```python
from build123d import *

# Parameters (mm, degrees)
SKETCH_1_R               = 17.5
EXTRUDE_1_DEPTH          = 25
EXTRUDE_2_DEPTH          = 9
SKETCH_3_R               = 9
EXTRUDE_3_DEPTH          = 3
CUT_EXTRUDE_1_DEPTH      = 49.736536602
CUT_EXTRUDE_1_DEPTH_BACK = 49.736536602
SKETCH_4_W               = 40.777628878
SKETCH_4_H               = 3
CUT_EXTRUDE_2_DEPTH      = 66.193941436
CUT_EXTRUDE_2_DEPTH_BACK = 66.193941436
SKETCH_5_R               = 10
CUT_EXTRUDE_3_REACH      = 56.215
SKETCH_6_R               = 5.5
HOLE_WIZARD_M10_1_D      = 8.5
SKETCH_9_W               = 16
SKETCH_9_H               = 50
EXTRUDE_4_DEPTH          = 41
SKETCH_10_W              = 82
SKETCH_10_H              = 10
EXTRUDE_5_DEPTH          = 8
EXTRUDE_6_DEPTH          = 4
EXTRUDE_7_DEPTH          = 20
SKETCH_13_R              = 14
CUT_EXTRUDE_4_DEPTH      = 3
SKETCH_14_R              = 7.5
CUT_EXTRUDE_5_DEPTH      = 153.663027613


with BuildPart() as part:
    # Sketch 1 → Extrude 1 (new, symmetric)
    with BuildSketch(Plane.XY):
        Circle(SKETCH_1_R)
    extrude(amount=EXTRUDE_1_DEPTH, both=True)

    # Sketch 2 → Extrude 2 (add, symmetric)
    with BuildSketch(Plane(origin=(0, 0, 0), x_dir=(1, 0, 0), z_dir=(0, 1, 0))):
        with BuildLine():
            Line((0, -13), (-25, -13))
            ThreePointArc((-25, -13), (-38, 0), (-25, 13))
            Line((-25, 13), (0, 13))
            ThreePointArc((0, 13), (13, 0), (0, -13))
        make_face()
    extrude(amount=EXTRUDE_2_DEPTH, both=True)

    # Sketch 3 → Extrude 3 (add)
    with BuildSketch(Plane(origin=(0, 9, 0), x_dir=(1, 0, 0), z_dir=(0, 1, 0))):
        with Locations(Location((-25, 0, 0), (0, 0, 270))):
            Circle(SKETCH_3_R)
    extrude(amount=EXTRUDE_3_DEPTH)

    # Sketch 4 → Cut-Extrude 1 (cut, two sides: drawn at the far end of the back side and taken through both)
    with BuildSketch(Plane.XY.offset(-CUT_EXTRUDE_1_DEPTH_BACK)):
        with Locations((-20.388814439, 0)):
            Rectangle(SKETCH_4_W, SKETCH_4_H)
    extrude(amount=CUT_EXTRUDE_1_DEPTH + CUT_EXTRUDE_1_DEPTH_BACK, mode=Mode.SUBTRACT)

    # Sketch 5 → Cut-Extrude 2 (cut, two sides: drawn at the far end of the back side and taken through both)
    with BuildSketch(Plane.XY.offset(25).offset(-CUT_EXTRUDE_2_DEPTH_BACK)):
        Circle(SKETCH_5_R)
    extrude(amount=CUT_EXTRUDE_2_DEPTH + CUT_EXTRUDE_2_DEPTH_BACK, mode=Mode.SUBTRACT)

    # Sketch 6 → Cut-Extrude 3 (cut, up to next)
    with BuildSketch(Plane(origin=(0, 12, 0), x_dir=(1, 0, 0), z_dir=(0, 1, 0)), mode=Mode.PRIVATE) as cut_extrude_3_sk1:
        with Locations(Location((-25, 0, 0), (0, 0, 270))):
            Circle(SKETCH_6_R)
    cut_extrude_3_tool1 = extrude(cut_extrude_3_sk1.sketch, amount=-CUT_EXTRUDE_3_REACH, mode=Mode.PRIVATE) & part.part
    add(cut_extrude_3_tool1.solids().sort_by_distance((-25, 12, 0))[0], mode=Mode.SUBTRACT)

    # Hole Wizard M10 _1 (through all)
    with Locations(Plane(origin=(0, -1.5, 0), x_dir=(1, 0, 0), z_dir=(0, 1, 0))):
        with Locations((-25, 0)):
            Hole(HOLE_WIZARD_M10_1_D / 2)



with BuildPart() as body_2:
    # Sketch 9 → Extrude 4 (new, symmetric)
    with BuildSketch(Plane.XY):
        with Locations((52, -95)):
            Rectangle(SKETCH_9_W, SKETCH_9_H)
    extrude(amount=EXTRUDE_4_DEPTH, both=True)

    # Sketch 10 → Extrude 5 (add)
    with BuildSketch(Plane(origin=(60, 0, 0), x_dir=(0, 0, -1), z_dir=(1, 0, 0))):
        with Locations((0, -75)):
            Rectangle(SKETCH_10_W, SKETCH_10_H)
    extrude(amount=EXTRUDE_5_DEPTH)


with BuildPart() as part_1:
    add(part.part)

    add(body_2.part)  # Extrude 6 merges body 2
    # Sketch 11 → Extrude 6 (add, symmetric)
    with BuildSketch(Plane.XY):
        with BuildLine():
            Line((-7, -16.039014932), (44, -115))
            Line((44, -115), (44, -70))
            Line((44, -70), (64, -70))
            Line((64, -70), (14.872506114, 9.222719875))
            ThreePointArc((14.872506114, 9.222719875), (13.229999981, -11.455003295), (-7, -16.039014932))
        make_face()
    extrude(amount=EXTRUDE_6_DEPTH, both=True)

    # Sketch 12 → Extrude 7 (add, symmetric)
    with BuildSketch(Plane.XY):
        with BuildLine():
            Line((64, -70), (14.872506114, 9.222719875))
            ThreePointArc((14.872506114, 9.222719875), (17.356401201, 2.237261127), (16.725134335, -5.149745768))
            Line((16.725134335, -5.149745768), (56.939992816, -70))
            Line((56.939992816, -70), (64, -70))
        make_face()
    extrude(amount=EXTRUDE_7_DEPTH, both=True)

    # Sketch 13 → Cut-Extrude 4 (cut)
    with BuildSketch(Plane.ZY.offset(-44)):
        with Locations(Location((-20, -100, 0), (0, 0, 270))):
            Circle(SKETCH_13_R)
    cut_extrude_4 = extrude(amount=-CUT_EXTRUDE_4_DEPTH, mode=Mode.SUBTRACT)

    # Sketch 14 → Cut-Extrude 5 (cut, through all)
    with BuildSketch(Plane.ZY.offset(-47)):
        with Locations(Location((-20, -100, 0), (0, 0, 270))):
            Circle(SKETCH_14_R)
    cut_extrude_5 = extrude(amount=-CUT_EXTRUDE_5_DEPTH, mode=Mode.SUBTRACT)

    # Mirror 1: Cut-Extrude 4, Cut-Extrude 5 across plane
    add(cut_extrude_4.mirror(Plane.XY), mode=Mode.SUBTRACT)
    add(cut_extrude_5.mirror(Plane.XY), mode=Mode.SUBTRACT)


solid = part_1.part
```
Check sheet for the modelled part. Datum: model origin and axes. Units: mm. A direction names the side the tool comes from. Round coordinates to 2 decimals unless told otherwise and drop trailing zeros. Loops run counter-clockwise (first coordinate to the right, second up) from the corner with the lowest first, then second, coordinate; pieces in that order, holes last. Notation, with made-up numbers: (76, 78.5) -> (101, 78.5) arc R18 cw to (101, 84.5) -> close; hole circle Ø6 at (-16, 65). An arc over 180 degrees is marked (long way). Write item = value, one per line. Start each with the question number.
1) Sectioned sample at A-A, the plane z = -18. Record the cut outline in (x, y), plus the area to 3 significant figures.
2) Sectioned sample at B-B, the plane x = 2.5. Record the cut outline in (y, z), plus the area to 3 significant figures.
3) Thickness scan on probe 1 along Z at (x, y) = (50.25, -100); probe 2 along Z at (x, y) = (46.3, -100); probe 3 along Y at (x, z) = (-25.5, 10.5). Record the ranges inside material, lowest first.
4) Set-up check for faces 1 (the flat face through (-34, 9, 3)), 2 (the flat face through (64, -80, 1)), 3 (the cylindrical face through (45.479, -112.932, -25.362)), 4 (the flat face through (36.55, -37.12, -11.89)): record each of +Z, -Z, +X, -X, +Y, -Y from which the full face is reachable in a straight line by a thin tool's end or side.
5) Sectioned sample at D-D, the plane x = 32.5. Record the cut outline in (y, z).
6) Release check for a two-part mould opening along Z. For faces 5 (the flat face through (53, -95, 41)), 6 (the flat face through (56, -70, 10)), 7 (the cylindrical face through (-19.547, 6.824, -0.716)), 8 (the flat face through (53, -95, -41)) record: released by +Z, released by -Z, zero draft, split by the parting line, or undercut.
7) Gauge pin test, flat ends, axial feed: pin 1 Ø4 at (y, z) = (-94, 2) entering from -X; pin 2 Ø2 at (x, z) = (49.5, -6) entering from +Y; pin 3 Ø25 at (y, z) = (-100, 20) entering from -X. Record the tip position at first contact, or that the pin passes through.
8) Sectioned sample at C-C, the plane y = -100. Record the cut outline in (x, z), plus the area to 3 significant figures.
Results are:
q1.outline = (-17.44, -1.5) arc R17.5 ccw to (16.73, -5.15) -> (56.94, -70) -> (44, -70) -> (44, -86.14) -> (47, -86.14) -> (47, -92.77) -> (60, -92.77) -> (60, -80) -> (68, -80) -> (68, -70) -> (64, -70) -> (14.87, 9.22) arc R17.5 ccw to (-17.44, 1.5) -> (-9.89, 1.5) arc R10 cw (long way) to (-9.89, -1.5) -> close; (44, -120) -> (60, -120) -> (60, -107.23) -> (47, -107.23) -> (47, -113.86) -> (44, -113.86) -> close
q1.area = 1,730 mm^2
q2.outline = (-34.47, -4) -> (-17.32, -4) -> (-17.32, -25) -> (-9.68, -25) -> (-9.68, 25) -> (-17.32, 25) -> (-17.32, 4) -> (-34.47, 4) -> close; (9.68, -25) -> (17.32, -25) -> (17.32, 25) -> (9.68, 25) -> close
q2.area = 901 mm^2
q3.probe_1 = -41 to -27.5, -12.5 to 12.5, 27.5 to 41
q3.probe_2 = -41 to -34, -6 to 6, 34 to 41
q3.probe_3 = -9 to -1.5, 1.5 to 9
q4.face_1 = +Y
q4.face_2 = +Z, -Z, +X, -Y
q4.face_3 = -X
q4.face_4 = -Z
q5.outline = (-92.69, -4) -> (-30.59, -4) -> (-30.59, -20) -> (-19.2, -20) -> (-19.2, 20) -> (-30.59, 20) -> (-30.59, 4) -> (-92.69, 4) -> close
q6.face_5 = released by +Z
q6.face_6 = zero draft
q6.face_7 = undercut
q6.face_8 = released by -Z
q7.pin_1 = 32.15
q7.pin_2 = -45
q7.pin_3 = 47
q8.outline = (36.27, -4) -> (44, -4) -> (44, -6) -> (47, -6) -> (47, -12.5) -> (60, -12.5) -> (60, 12.5) -> (47, 12.5) -> (47, 6) -> (44, 6) -> (44, 4) -> (36.27, 4) -> close; (44, -41) -> (60, -41) -> (60, -27.5) -> (47, -27.5) -> (47, -34) -> (44, -34) -> close; (44, 34) -> (47, 34) -> (47, 27.5) -> (60, 27.5) -> (60, 41) -> (44, 41) -> close
q8.area = 816 mm^2
